Design review of the part built by this model. Coordinates are the model's own, in mm. Face numbers are marked on the shaded views. Round coordinates to 2 decimals unless told otherwise and drop trailing zeros. Order: outer loops, then holes, each group sorted by start corner. A loop starts at its lowest first (then second) coordinate and runs counter-clockwise, first axis right, second up. Notation, with made-up numbers: M -16,82.25 L 6,82.25 A14 cw 6,96.25 Z; hole C 25,37 d4. An arc over 180 degrees is marked long. Write each question's results on one line, items separated by ' | '. Start each with the question number.
Item 1: Take a section at A-A, the plane y = 5.5. Write out the cut boundary in (x, z).
Item 2: Clearance check with a flat-ended pin moving along its axis: pin 1 (1.8 mm diameter, centred on x = 15, y = 5.5, fed in from +Z). State where the tip first meets the part, or that it passes through.
Item 3: Take a section at C-C, the plane x = 15. Write out the cut boundary in (y, z), plus the area to 4 significant figures.
Item 4: Wall thickness on line 1 (X direction, y = 5.75, z = 2.8); line 2 (Y direction, x = 15, z = 1); line 3 (Y direction, x = 16, z = 3.05): over which ranges is each line inside the solid? List them lowest first. Write a range as [from, to].
Item 5: The part is to be moulded in two halves that separate along X. For the marked faces 1, 2, 3 and 4, say which applies: +X half, -X half, draft (parallel to the pull), parting line (faces both ways), or undercut.
Item 6: Take a section at B-B, the plane z = 1.4. Write out the cut boundary in (x, y), plus the area to 3 significant figures.
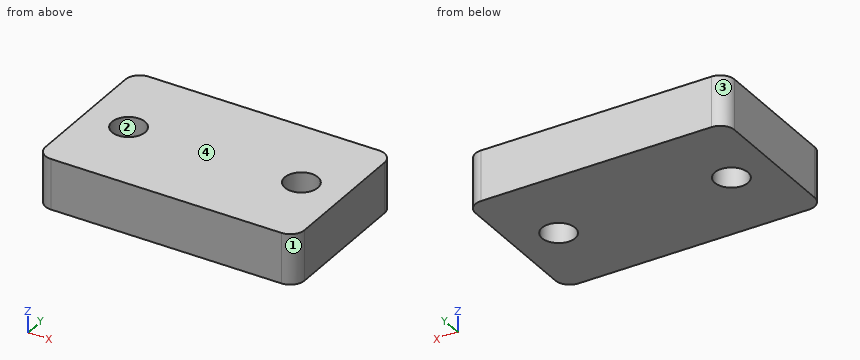
```python
from build123d import *

# Parameters (mm, degrees)
SKETCH_1_W      = 18
SKETCH_1_H      = 11
SKETCH_1_R      = 1.15
EXTRUDE_1_DEPTH = 3.5
FILLET_1_R      = 1


with BuildPart() as part:
    # 草图1 → 凸台-拉伸1 (new body)
    with BuildSketch(Plane.XY):
        with Locations((9, 5.5)):
            Rectangle(SKETCH_1_W, SKETCH_1_H)
        with Locations((3, 5.5)):
            Circle(SKETCH_1_R, mode=Mode.SUBTRACT)
        with Locations((15, 5.5)):
            Circle(SKETCH_1_R, mode=Mode.SUBTRACT)
    extrude(amount=EXTRUDE_1_DEPTH)

    # 圆角1
    fillet_1_edges = [part.edges().sort_by_distance(p)[0] for p in [
        (0, 11, 1.75),
        (18, 11, 1.75),
        (18, 0, 1.75),
        (0, 0, 1.75),
    ]]
    fillet(fillet_1_edges, radius=FILLET_1_R)


solid = part.part
```
Results list:
1) outline: M 0,0 L 1.85,0 L 1.85,3.5 L 0,3.5 Z; M 4.15,0 L 13.85,0 L 13.85,3.5 L 4.15,3.5 Z; M 16.15,0 L 18,0 L 18,3.5 L 16.15,3.5 Z
2) pin 1: through
3) outline: M 0,0 L 4.35,0 L 4.35,3.5 L 0,3.5 Z; M 6.65,0 L 11,0 L 11,3.5 L 6.65,3.5 Z | area: 30.45 mm²
4) line 1: [0, 1.88], [4.12, 13.88], [16.12, 18] | line 2: [0, 4.35], [6.65, 11] | line 3: [0, 4.93], [6.07, 11]
5) face 1: +X half | face 2: undercut | face 3: -X half | face 4: draft
6) outline: M 0,1 A1 ccw 1,0 L 17,0 A1 ccw 18,1 L 18,10 A1 ccw 17,11 L 1,11 A1 ccw 0,10 Z; hole C 3,5.5 d2.3; hole C 15,5.5 d2.3 | area: 189 mm²
